Can you work these out from the drawing? Everything is in mm from the part's minimum corner. Coordinates: 2 decimals unless noted, no trailing zeros. Write each loop counter-clockwise with the first axis right and the second up, starting at its lowest first coordinate (ties: lowest second). Pieces come first, ordered by that corner, then holes.
(1) Imagine slicing it at D-D, the plane x = 35. List the corners of the cut face in (y, z) for me, plus the area to 3 significant figures.
(2) Imagine slicing it at B-B, the plane z = 27.5. List the corners of the cut face in (x, y) for me.
(3) Imagine slicing it at C-C, the plane z = 3.5. List the corners of the cut face in (x, y) for me.
(4) Please list where these lines run through material, in increasing order: probe 1 along Z at (x, y) = (26.5, 1.8); probe 2 along X at (y, z) = (1.55, 31); probe 3 along X at (y, z) = (0.1, 24.5).
(5) Imagine slicing it at A-A, the plane y = 0.8. List the corners of the cut face in (x, z) for me.
(6) For pin 1 Ø3 at (x, z) = (5.5, 48) entering from -Y; pin 2 Ø3 at (x, z) = (23, 3.5) entering from +Y, each with a flat end and sliding along its axis, tell me the tip position at first contact or that it passes through.
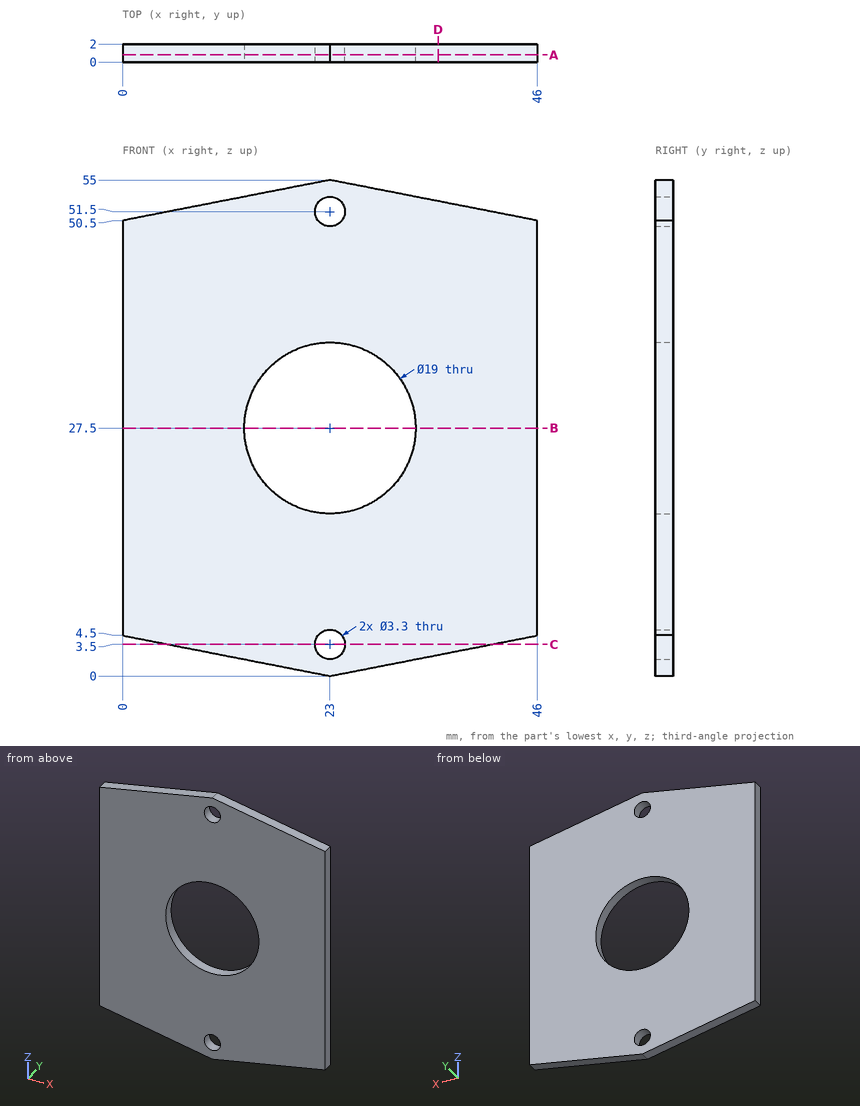
Recorded:
1. outline: (0, 2.35) - (2, 2.35) - (2, 52.65) - (0, 52.65) - close
1. area: 101 mm2
2. outline: (0, 0) - (13.5, 0) - (13.5, 2) - (0, 2) - close; (32.5, 0) - (46, 0) - (46, 2) - (32.5, 2) - close
3. outline: (5.11, 0) - (21.35, 0) - (21.35, 2) - (5.11, 2) - close; (24.65, 0) - (40.89, 0) - (40.89, 2) - (24.65, 2) - close
4. probe 1: z = 0.68 to 18.67, 36.33 to 54.32
4. probe 2: x = 0 to 14.17, 31.83 to 46
4. probe 3: x = 0 to 13.99, 32.01 to 46
5. outline: (0, 4.5) - (23, 0) - (46, 4.5) - (46, 50.5) - (23, 55) - (0, 50.5) - close; hole circle Ø19 at (23, 27.5); hole circle Ø3.3 at (23, 3.5); hole circle Ø3.3 at (23, 51.5)
6. pin 1: stops at y = 0
6. pin 2: passes through
